Build history of the part. All positions in model axes, mm. A direction names the side the tool comes from. Round coordinates to 2 decimals unless told otherwise and drop trailing zeros. Order: outer loops, then holes, each group sorted by start corner. A loop starts at its lowest first (then second) coordinate and runs counter-clockwise, first axis right, second up. Notation, with made-up numbers: M 36.25,68 L 74.25,68 A16 ccw 74.25,99 Z; hole C 83,82.25 d4. An arc over 180 degrees is marked long. One line per item, written item: value. Start each with the question number.
Item 1: Band-saw the part on B-B, the plane y = 2.75. Write the cut outline in (x, z), then the cut area to 3 significant figures.
Item 2: Pin check, flat tips, straight feed: pin 1 (3 mm diameter, centred on x = 0, z = 2, fed in from -Y); pin 2 (1.1 mm diameter, centred on x = 0.5, z = 0, fed in from +Y); pin 3 (1 mm diameter, centred on y = -1.5, z = 3.5, fed in from -X); pin 4 (2 mm diameter, centred on x = -8, y = -4, fed in from -Z). Stop position of each tip, or through.
Item 3: Tool access for faces 5 (the cylindrical face through (-3.47, 9.49, 1.16)), 6 (the cylindrical face through (3.47, -9.49, 1.16)), 7 (the flat face through (2.737, -1.61, 1.162)), 8 (the cylindrical face through (5.54, -9.626, 1.162)): list every direction of +Z, -Z, +X, -X, +Y, -Y with a clear straight run to the whole face (end or side of a thin tool).
Item 4: Band-saw the part on C-C, the plane x = 7.25. Write the cut outline in (y, z).
Item 5: Probe L1, parallel to Y at x = 0, z = -0.5 (3 decimals); L2, parallel to X at y = 3, z = 1; L3, parallel to Y at x = -8.75, z = 3.25. List the from-to ranges inside material, lowest first.
Item 6: Band-saw the part on A-A, the plane x = 0.5. Write the cut outline in (y, z) (3 decimals).
Item 7: Two-plate mould, pull along Y, no slides. Class faces 1 (the cylindrical face through (6.49, -7.78, 1.16)), 2 (the flat face through (2.76, 1.57, 1.16)), 3 (the cylindrical face through (9.95, -1.743, 1.162)), 4 (the cylindrical face through (-5.54, 9.626, 1.162)): +Y half, -Y half, draft (parallel to the pull), parting line (faces both ways), or undercut.
```python
from build123d import *

# Parameters (mm, degrees)
BOSS_EXTRUDE1_DEPTH = 6.35
CUT_EXTRUDE1_DEPTH  = 17.308131721


with BuildPart() as part:
    # Sketch1 → Boss-Extrude1 (new body)
    with BuildSketch(Plane.XY.offset(4.2926)):
        with BuildLine():
            Line((-6.148414016, 6.539673115), (-6.079307951, 6.381995928))
            ThreePointArc((-6.079307951, 6.381995928), (-5.900367293, 5.91212738), (-5.757411872, 5.43009008))
            ThreePointArc((-5.757411872, 5.43009008), (-6.015092025, 3.472815), (-7.581301891, 2.271019901))
            ThreePointArc((-7.581301891, 2.271019901), (-8.070236148, 2.153804277), (-8.566624576, 2.073837159))
            Line((-8.566624576, 2.073837159), (-8.737730058, 2.054846173))
            ThreePointArc((-8.737730058, 2.054846173), (-9.966107592, 1.73564362), (-11.053625442, 1.081345092))
            ThreePointArc((-11.053625442, 1.081345092), (-11.106391971, 0), (-11.053625442, -1.081345092))
            ThreePointArc((-11.053625442, -1.081345092), (-9.966107592, -1.73564362), (-8.737730058, -2.054846173))
            Line((-8.737730058, -2.054846173), (-8.566624576, -2.073837159))
            ThreePointArc((-8.566624576, -2.073837159), (-8.070236148, -2.153804277), (-7.581301891, -2.271019901))
            ThreePointArc((-7.581301891, -2.271019901), (-6.015092025, -3.472815), (-5.757411872, -5.43009008))
            ThreePointArc((-5.757411872, -5.43009008), (-5.900367293, -5.91212738), (-6.079307951, -6.381995928))
            Line((-6.079307951, -6.381995928), (-6.148414016, -6.539673115))
            ThreePointArc((-6.148414016, -6.539673115), (-6.486165263, -7.763080542), (-6.463285041, -9.03204789))
            ThreePointArc((-6.463285041, -9.03204789), (-5.553195986, -9.618417591), (-4.590340401, -10.113392982))
            ThreePointArc((-4.590340401, -10.113392982), (-3.479942329, -9.498724162), (-2.589316042, -8.594519288))
            Line((-2.589316042, -8.594519288), (-2.487316625, -8.455833087))
            ThreePointArc((-2.487316625, -8.455833087), (-2.169868855, -8.065931658), (-1.823890018, -7.701109982))
            ThreePointArc((-1.823890018, -7.701109982), (0, -6.94563), (1.823890018, -7.701109982))
            ThreePointArc((1.823890018, -7.701109982), (2.169868855, -8.065931658), (2.487316625, -8.455833087))
            Line((2.487316625, -8.455833087), (2.589316042, -8.594519288))
            ThreePointArc((2.589316042, -8.594519288), (3.479942329, -9.498724162), (4.590340401, -10.113392982))
            ThreePointArc((4.590340401, -10.113392982), (5.553195986, -9.618417591), (6.463285041, -9.03204789))
            ThreePointArc((6.463285041, -9.03204789), (6.486165263, -7.763080542), (6.148414016, -6.539673115))
            Line((6.148414016, -6.539673115), (6.079307951, -6.381995928))
            ThreePointArc((6.079307951, -6.381995928), (5.900367293, -5.91212738), (5.757411872, -5.43009008))
            ThreePointArc((5.757411872, -5.43009008), (6.015092025, -3.472815), (7.581301891, -2.271019901))
            ThreePointArc((7.581301891, -2.271019901), (8.070236148, -2.153804277), (8.566624576, -2.073837159))
            Line((8.566624576, -2.073837159), (8.737730058, -2.054846173))
            ThreePointArc((8.737730058, -2.054846173), (9.966107592, -1.73564362), (11.053625442, -1.081345092))
            ThreePointArc((11.053625442, -1.081345092), (11.106391971, 0), (11.053625442, 1.081345092))
            ThreePointArc((11.053625442, 1.081345092), (9.966107592, 1.73564362), (8.737730058, 2.054846173))
            Line((8.737730058, 2.054846173), (8.566624576, 2.073837159))
            ThreePointArc((8.566624576, 2.073837159), (8.070236148, 2.153804277), (7.581301891, 2.271019901))
            ThreePointArc((7.581301891, 2.271019901), (6.015092025, 3.472815), (5.757411872, 5.43009008))
            ThreePointArc((5.757411872, 5.43009008), (5.900367293, 5.91212738), (6.079307951, 6.381995928))
            Line((6.079307951, 6.381995928), (6.148414016, 6.539673115))
            ThreePointArc((6.148414016, 6.539673115), (6.486165263, 7.763080542), (6.463285041, 9.03204789))
            ThreePointArc((6.463285041, 9.03204789), (5.553195986, 9.618417591), (4.590340401, 10.113392982))
            ThreePointArc((4.590340401, 10.113392982), (3.479942329, 9.498724162), (2.589316042, 8.594519288))
            Line((2.589316042, 8.594519288), (2.487316625, 8.455833087))
            ThreePointArc((2.487316625, 8.455833087), (2.169868855, 8.065931658), (1.823890018, 7.701109982))
            ThreePointArc((1.823890018, 7.701109982), (0, 6.94563), (-1.823890018, 7.701109982))
            ThreePointArc((-1.823890018, 7.701109982), (-2.169868855, 8.065931658), (-2.487316625, 8.455833087))
            Line((-2.487316625, 8.455833087), (-2.589316042, 8.594519288))
            ThreePointArc((-2.589316042, 8.594519288), (-3.479942329, 9.498724162), (-4.590340401, 10.113392982))
            ThreePointArc((-4.590340401, 10.113392982), (-5.553195986, 9.618417591), (-6.463285041, 9.03204789))
            ThreePointArc((-6.463285041, 9.03204789), (-6.486165263, 7.763080542), (-6.148414016, 6.539673115))
        make_face()
    extrude(amount=-BOSS_EXTRUDE1_DEPTH)

    # Sketch2 → Cut-Extrude1 (cut, through all)
    with BuildSketch(Plane.XY.offset(4.2926)):
        Polygon((3.666174209, 0), (1.833087105, 3.175), (-1.833087105, 3.175), (-3.666174209, 0), (-1.833087105, -3.175), (1.833087105, -3.175), align=None)
    extrude(amount=-CUT_EXTRUDE1_DEPTH, mode=Mode.SUBTRACT)


solid = part.part
```
Output:
1. outline: M -6.64,-2.06 L -2.08,-2.06 L -2.08,4.29 L -6.64,4.29 Z; M 2.08,-2.06 L 6.64,-2.06 L 6.64,4.29 L 2.08,4.29 Z
1. area: 57.9 mm²
2. pin 1: stops at y = -7.43
2. pin 2: stops at y = 7.17
2. pin 3: stops at x = -11.06
2. pin 4: passes through
3. face 5: +Z, -Z, +Y
3. face 6: +Z, -Z, -Y
3. face 7: +Z, -Z
3. face 8: +Z, -Z, +X, -Y
4. outline: M -2.38,-2.06 L 2.38,-2.06 L 2.38,4.29 L -2.38,4.29 Z
5. L1: y = -6.946 to -3.175, 3.175 to 6.946
5. L2: x = -6.37 to -1.93, 1.93 to 6.37
5. L3: y = -2.05 to 2.05
6. outline: M -6.995,-2.057 L -3.175,-2.057 L -3.175,4.293 L -6.995,4.293 Z; M 3.175,-2.057 L 6.995,-2.057 L 6.995,4.293 L 3.175,4.293 Z
7. face 1: undercut
7. face 2: undercut
7. face 3: -Y half
7. face 4: +Y half
